Autodesk Inventor part; units mm, degrees
ref_plane "YZ Plane" through (0, 0, 0) normal (1, 0, 0) x (0, 1, 0)
ref_plane "XZ Plane" through (0, 0, 0) normal (0, 1, 0) x (-1, 0, 0)
ref_plane "XY Plane" through (0, 0, 0) normal (0, 0, 1) x (1, 0, 0)
sketch "Sketch1" plane through (0, 0, 0) normal (0, 1, 0) x (-1, 0, 0)
  line L0 (0, 0) -> (0, -125.2474)
  line L1 (0, -125.2474) -> (-3.4036, -125.2474)
  line L2 (0, 0) -> (-3.4036, 0)
  line L3 (-3.4036, 0) -> (-0.889, -31.2039)
  line L4 (-0.889, -31.2039) -> (-6.5786, -62.4078)
  line L5 (-6.5786, -62.4078) -> (-0.889, -94.0308)
  line L6 (-0.889, -94.0308) -> (-3.4036, -125.2474)
  dimension "d0" = 125.2474
  dimension "d1" = 3.4036
  dimension "d2" = 3.4036
  dimension "d3" = 31.2039
  dimension "d4" = 62.4078
  dimension "d5" = 31.2166
  dimension "d15" = 6.5786
  dimension "d16" = 0.889
  dimension "d17" = 0.889
extrude "Extrusion1" add sketch "Sketch1" along normal blind 5.8166
sketch "Sketch2" plane through (0, 0, 0) normal (0, 0, 1) x (1, 0, 0)
  line L0 (3.4036, 0) -> (0, 0)
  line L1 (0, 5.8166) -> (1.651, 5.8166)
  line L2 (1.651, 5.8166) -> (1.651, 0)
  line L3 (1.651, 0) -> (0, 0)
  line L4 (0, 0) -> (0, 5.8166)
  dimension "d8" = 1.651
sketch "Sketch3" plane through (3.4036, 0, -125.2474) normal (0, 0, -1) x (-1, 0, 0)
  line L0 (3.4036, 0) -> (3.4036, 5.8166)
  line L1 (0, 0) -> (3.4036, 0)
  line L2 (3.4036, 5.8166) -> (1.7526, 5.8166)
  line L3 (1.7526, 5.8166) -> (1.7526, 0)
  line L4 (1.7526, 0) -> (3.4036, 0)
  line L5 (3.4036, 0) -> (3.4036, 5.8166)
  dimension "d9" = 1.651
extrude "Extrusion2" add sketch "Sketch3" along normal blind 2.5654
extrude "Extrusion3" add sketch "Sketch2" along normal blind 2.5654
properties part number "long_insert_inv_CPY"
Geometry: final body of the model. Coordinates: model frame, mm. A direction names the side the tool comes from. Round coordinates to 2 decimals unless told otherwise and drop trailing zeros. Write each loop counter-clockwise with the first axis right and the second up, starting at its lowest first coordinate (ties: lowest second). Pieces come first, ordered by that corner, then holes. Notation, with made-up numbers: (76, -30) -> (132, -30) arc R30 ccw to (132, 5) -> close; hole circle Ø2 at (72, 17). An arc over 180 degrees is marked (long way). Use CSV: the item, a comma, the result in double quotes. Start each with the question number.
Q1. Section A-A (y = 2.45). Return loops of the section in (x, z), plus the area to 3 significant figures.
Q2. Section C-C (x = 4.5). Return loops of the section in (y, z).
Q3. First-contact query: pin 1 Ø0.8 at (y, z) = (3, 1.5) entering from +X; pin 2 Ø1.4 at (x, y) = (2.5, 2) entering from +Z; pin 3 Ø1.4 at (x, y) = (2.5, 3) entering from -Z. Flat tips, straight axial feed; report the tip coordinate or a pass-through.
Q4. Line query: L1, parallel to X at y = 4.2, z = -51; L2, parallel to X at y = 0.6, z = -12. Output: solid intervals per line, ascending.
Q5. Pull-direction query (Z, two-part tool) for faces 4 (the face through (1.651, 3, -127)), 5 (the face through (3.694, 2.868, -46.587)); classes: pulls with the +Z half, pulls with the -Z half, needs draft (parallel to the pull), parting line crosses it, or undercut.
Q6. Reachability of faces 1 (the face through (1.651, 3, 1)), 2 (the face through (0, 3, -64)), 3 (the face through (2.164, 2.868, -15.384)) from +Z, -Z, +X, -X, +Y, -Y: full face, straight path, thin tool, end or side. Return the list, or none.
Q7. Section B-B (z = -88). Return loops of the section in (x, y), plus the area to 3 significant figures.
Result sheet:
1,outline,"(0, -127.81) -> (1.65, -127.81) -> (1.65, -125.25) -> (3.4, -125.25) -> (0.89, -94.03) -> (6.58, -62.41) -> (0.89, -31.2) -> (3.4, 0) -> (1.65, 0) -> (1.65, 2.57) -> (0, 2.57) -> close"
1,area,"377 mm²"
2,outline,"(0, -73.96) -> (5.82, -73.96) -> (5.82, -51.01) -> (0, -51.01) -> close"
3,pin 1,"x = 1.65"
3,pin 2,"z = 0"
3,pin 3,"z = -125.25"
4,L1,"0 to 4.5"
4,L2,"0 to 2.44"
5,face 4,"needs draft"
5,face 5,"undercut"
6,face 1,"+Z, +X, +Y, -Y"
6,face 2,"+Z, -Z, -X, +Y, -Y"
6,face 3,"+X, +Y, -Y"
7,outline,"(0, 0) -> (1.97, 0) -> (1.97, 5.82) -> (0, 5.82) -> close"
7,area,"11.5 mm²"
